For this review, use the dimensioned drawing (mm, ordinates from the lowest corner) and the shaded views. A direction names the side the tool comes from. Coordinates: 2 decimals unless noted, no trailing zeros. Loops run counter-clockwise (first coordinate to the right, second up) from the corner with the lowest first, then second, coordinate; pieces in that order, holes last. Notation, with made-up numbers: M 7,17 L 38,17 A24 cw 38,38 Z; hole C 60.5,37 d7. An arc over 180 degrees is marked long. One line per item, written item: value.
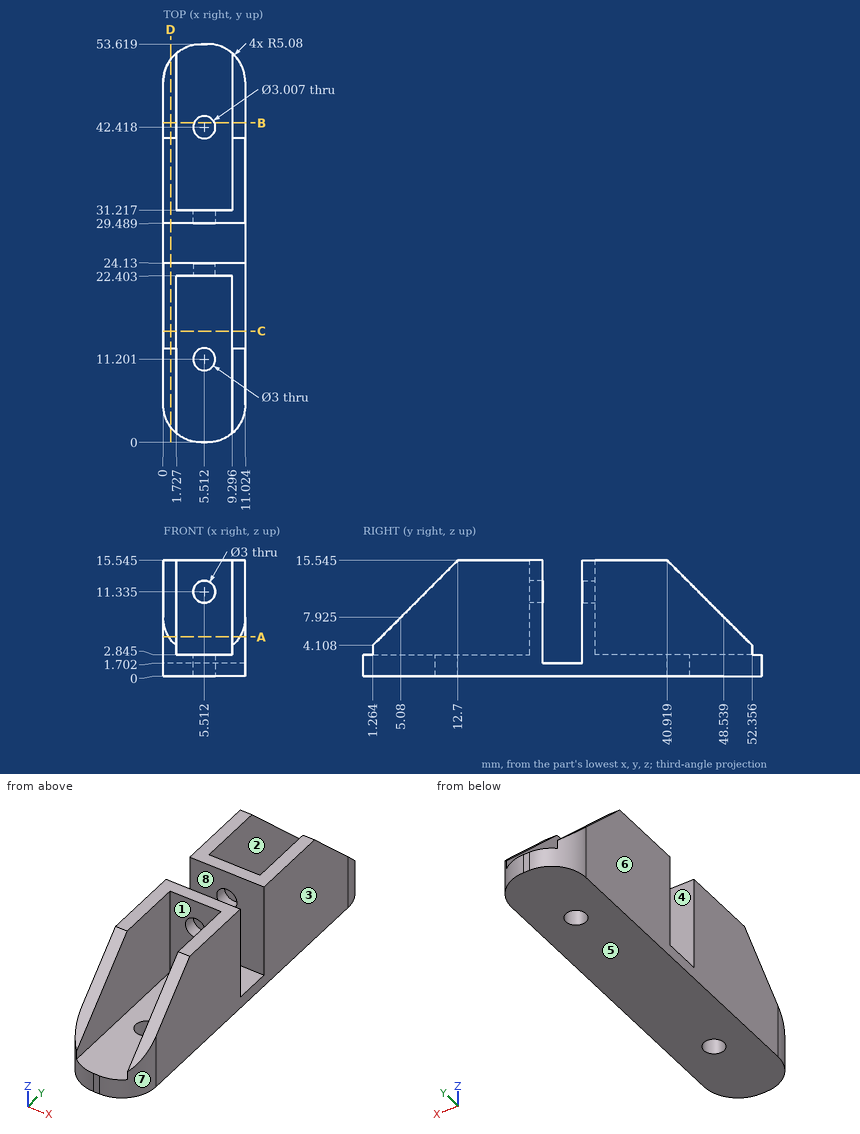
(1) Add section B-B on y = 43. State the section outline as (x, z) points (1 decimal).
Checks:
outline: M 0,0 L 4.1,0 L 4.1,2.8 L 1.7,2.8 L 1.7,13.5 L 0,13.5 Z; M 6.9,0 L 11,0 L 11,13.5 L 9.3,13.5 L 9.3,2.8 L 6.9,2.8 Z
(2) To check wall thickness, follow L1, parallel to X at y = 42.5, z = 8.5; L2, parallel to Y at x = 7.25, z = 12.5; L3, parallel to Z at x = 7, y = 27. State the ranges of each line that lie inside material, in increasing order. Write a range as [from, to].
Checks:
L1: [0, 1.73], [9.3, 11.02]
L2: [22.4, 24.13], [29.49, 31.22]
L3: [0, 1.7]
(3) Draft analysis for pull direction Y (two halves, no side actions). For the marked faces 6, 7 and 8, state which applies: pulls with the +Y half, pulls with the -Y half, needs draft (parallel to the pull), parting line crosses it, or undercut.
Checks:
face 6: needs draft
face 7: pulls with the -Y half
face 8: undercut
(4) Insertion check: pin 1 Ø6 at (x, y) = (4, 41) entering from +Z (1 decimal); pin 2 Ø6 at (x, z) = (2, 13.5) entering from +Y; pin 3 Ø2.5 at (x, z) = (5.51, 11.33) entering from -Y; pin 4 Ø5 at (x, y) = (5.51, 42.42) entering from +Z (1 decimal). Each pin has a flat end and moves straight along its axis. Give the tip position at first contact, or say it passes through.
Checks:
pin 1: z = 15.5
pin 2: y = 45.95
pin 3: through
pin 4: z = 2.8
(5) Add section C-C on y = 15. State the section outline as (x, z) points (1 decimal).
Checks:
outline: M 0,0 L 11,0 L 11,15.5 L 9.3,15.5 L 9.3,2.8 L 1.7,2.8 L 1.7,15.5 L 0,15.5 Z
(6) Add section D-D on x = 1. State the section outline as (y, z) points (1 decimal), then the cut area to 3 significant figures.
Checks:
outline: M 2.1,0 L 51.6,0 L 51.6,4.9 L 40.9,15.5 L 29.5,15.5 L 29.5,1.7 L 24.1,1.7 L 24.1,15.5 L 12.7,15.5 L 2.1,4.9 Z
area: 582 mm^2
(7) Add section A-A on z = 5.25. State the section outline as (x, y) points (1 decimal).
Checks:
outline: M 0,5.1 A5.1 ccw 0.8,2.4 L 1.7,2.4 L 1.7,22.4 L 9.3,22.4 L 9.3,2.4 L 10.3,2.4 A5.1 ccw 11,5.1 L 11,24.1 L 0,24.1 Z; M 0,29.5 L 11,29.5 L 11,48.5 A5.1 ccw 10.3,51.2 L 9.3,51.2 L 9.3,31.2 L 1.7,31.2 L 1.7,51.2 L 0.8,51.2 A5.1 ccw 0,48.5 Z
(8) Tool access review of the marked faces 1, 2, 3, 4 and 5: name each direction out of +Z, -Z, +X, -X, +Y, -Y from which nothing blocks a thin tool from reaching the whole face with its end or side.
Checks:
face 1: +Z, -Y
face 2: +Z, +Y
face 3: +Z, -Z, +X, +Y, -Y
face 4: +Z, +X, -X
face 5: -Z, +X, -X, +Y, -Y
